```python
from build123d import *

# Parameters (mm, degrees)
SKETCH3_W           = 50
SKETCH3_H           = 50
BOSS_EXTRUDE1_DEPTH = 1.5875
BOSS_EXTRUDE2_DEPTH = 0.204346
SKETCH4_W           = 10
SKETCH4_H           = 10
BOSS_EXTRUDE3_DEPTH = 0.675
SKETCH5_W           = 0.9
SKETCH5_H           = 0.3
BOSS_EXTRUDE4_DEPTH = 0.001


with BuildPart() as part:
    # Sketch3 → Boss-Extrude1 (new body)
    with BuildSketch(Plane(origin=(0, 0, 0), x_dir=(1, 0, 0), z_dir=(0, 1, 0))):
        with Locations((22.488763021, 23.818655395)):
            Rectangle(SKETCH3_W, SKETCH3_H)
    extrude(amount=-BOSS_EXTRUDE1_DEPTH)

    # Sketch2 → Boss-Extrude2 (add)
    with BuildSketch(Plane(origin=(0, 0, 0), x_dir=(1, 0, 0), z_dir=(0, 1, 0))):
        Polygon((32.488763021, 28.302249005), (32.488763021, 40.851579566), (47.488763021, 48.818655395), (-2.511236979, 48.818655395), (12.488763021, 40.851579566), (12.488763021, 28.302249005), align=None)
        Polygon((47.488763021, 31.033343899), (47.488763021, 36.033343899), (42.488763021, 36.033343899), (40.243873607, 34.239185764), (35.010861347, 34.239185764), (35.010861347, 27.818655395), (19.338763021, 27.818655395), (19.338763021, 27.518655395), (36.72925203, 27.518655395), (36.72925203, 32.827502034), (40.243873607, 32.827502034), (42.488763021, 31.033343899), align=None)
        Polygon((47.488763021, -1.181344605), (47.488763021, 3.818655395), (45.72925203, 6.01706342), (45.72925203, 26.536834752), (25.338763021, 26.536834752), (25.338763021, 26.818655395), (25.038763021, 26.818655395), (25.038763021, 26.236834752), (41.093092119, 26.236834752), (44.248274012, 23.081652859), (44.248274012, 6.01706342), (42.488763021, 3.818655395), (42.488763021, -1.181344605), align=None)
        Polygon((33.488763021, -1.181344605), (38.488763021, -1.181344605), (38.488763021, 3.818655395), (36.72925203, 6.01706342), (36.72925203, 24.975395702), (24.138763021, 24.975395702), (24.138763021, 26.818655395), (23.838763021, 26.818655395), (23.838763021, 24.686834752), (33.643092119, 24.686834752), (35.248274012, 23.081652859), (35.248274012, 6.01706342), (33.488763021, 3.818655395), align=None)
        Polygon((24.488763021, 3.818655395), (24.488763021, -1.181344605), (29.488763021, -1.181344605), (29.488763021, 3.818655395), (27.72925203, 6.01706342), (27.72925203, 23.436834752), (22.938763021, 23.436834752), (22.938763021, 26.818655395), (22.638763021, 26.818655395), (22.638763021, 23.136834752), (24.213594494, 23.136834752), (26.248274012, 21.102155233), (26.248274012, 6.01706342), align=None)
        Polygon((15.488763021, 3.818655395), (15.488763021, -1.181344605), (20.488763021, -1.181344605), (20.488763021, 3.818655395), (18.72925203, 6.01706342), (18.731288885, 21.102155233), (20.765968404, 23.136834752), (21.738763021, 23.136834752), (21.738763021, 26.818655395), (21.438763021, 26.818655395), (21.438763021, 23.436834752), (17.248274012, 23.436834752), (17.248274012, 6.01706342), align=None)
        Polygon((6.488763021, 3.818655395), (6.488763021, -1.181344605), (11.488763021, -1.181344605), (11.488763021, 3.818655395), (9.732070762, 6.01706342), (9.732070762, 23.081652859), (11.325813604, 24.686834752), (20.538763021, 24.686834752), (20.538763021, 26.818655395), (20.238763021, 26.818655395), (20.238763021, 24.986834752), (8.24545528, 24.986834752), (8.24545528, 6.01706342), align=None)
        Polygon((-0.735853149, 6.01706342), (-2.511236979, 3.818655395), (-2.511236979, -1.181344605), (2.488763021, -1.181344605), (2.488763021, 3.818655395), (0.729267736, 6.01706342), (0.729267736, 23.081652859), (3.884449629, 26.236834752), (19.338763021, 26.236834752), (19.338763021, 26.818655395), (19.038763021, 26.818655395), (19.038763021, 26.536834752), (-0.735853149, 26.536834752), align=None)
    extrude(amount=BOSS_EXTRUDE2_DEPTH)

    # Sketch4 → Boss-Extrude3 (add)
    with BuildSketch(Plane(origin=(0, 0.204346, 0), x_dir=(1, 0, 0), z_dir=(0, 1, 0))):
        with Locations((22.488763021, 33.818655395)):
            Rectangle(SKETCH4_W, SKETCH4_H)
    extrude(amount=BOSS_EXTRUDE3_DEPTH)

    # Sketch5 → Boss-Extrude4 (add)
    with BuildSketch(Plane(origin=(0, 0.879346, 0), x_dir=(1, 0, 0), z_dir=(0, 1, 0))):
        with Locations((19.488763021, 30.118655395)):
            Rectangle(SKETCH5_W, SKETCH5_H)
        with Locations((20.688763021, 30.118655395)):
            Rectangle(SKETCH5_W, SKETCH5_H)
        with Locations((21.888763021, 30.118655395)):
            Rectangle(SKETCH5_W, SKETCH5_H)
        with Locations((23.088763021, 30.118655395)):
            Rectangle(SKETCH5_W, SKETCH5_H)
        with Locations((24.288763021, 30.118655395)):
            Rectangle(SKETCH5_W, SKETCH5_H)
        with Locations((25.488763021, 30.118655395)):
            Rectangle(SKETCH5_W, SKETCH5_H)
    extrude(amount=BOSS_EXTRUDE4_DEPTH)


solid = part.part
```
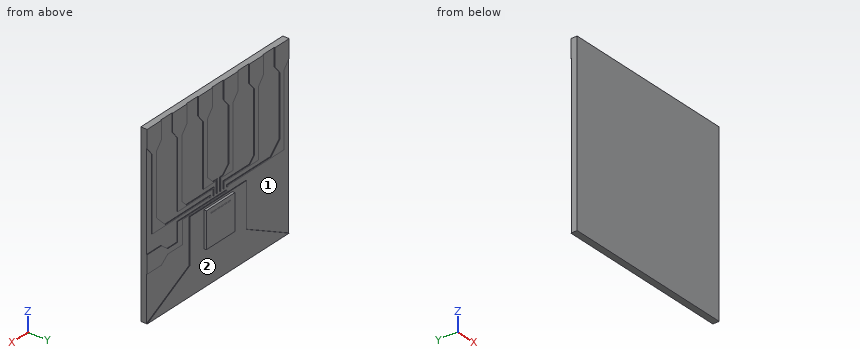
Check sheet for the modelled part. Datum: model origin and axes. Units: mm. Face numbers are marked on the shaded views. Coordinates: 2 decimals unless noted, no trailing zeros. Loops run counter-clockwise (first coordinate to the right, second up) from the corner with the lowest first, then second, coordinate; pieces in that order, holes last. Notation, with made-up numbers: M -25.5,-36 L 0.5,-36 A19 ccw 0.5,-7 Z; hole C 15.25,21.5 d1. An arc over 180 degrees is marked long. Answer as a JSON object with one key per item and string values.
1. Depth check by flat-ended pin: P1, Ø7, axis at x = 13.5, z = -17.5, coming from the +Y side; P2, Ø5.5, axis at x = 25, z = -13, coming from the +Y side; P3, Ø10, axis at x = 25.5, z = -28, coming from the +Y side. Enter the tip coordinate at first touch or a pass-through.
Outcome:
{"P1": "y = 0", "P2": "y = 0.2", "P3": "y = 0.88"}
2. Release check for a two-part mould opening along Z. For the marked faces 1 and 2 record: pulls with the +Z half, pulls with the -Z half, needs draft (parallel to the pull), parting line crosses it, or undercut.
Outcome:
{"face 1": "undercut", "face 2": "needs draft"}
3. Sectioned sample at A-A on x = 37.5. Record the cut outline in (y, z), and give its area (3 significant figures).
Outcome:
{"outline": "M -1.59,-48.82 L 0.2,-48.82 L 0.2,-43.51 L 0,-43.51 L 0,-34.24 L 0.2,-34.24 L 0.2,-32.83 L 0,-32.83 L 0,-26.54 L 0.2,-26.54 L 0.2,-26.24 L 0,-26.24 L 0,-5.05 L 0.2,-5.05 L 0.2,1.18 L -1.59,1.18 Z", "area": "82.1 mm²"}
4. Sectioned sample at B-B on z = -18. Record the cut outline in (x, y), and give its area (3 significant figures).
Outcome:
{"outline": "M -2.51,-1.59 L 47.49,-1.59 L 47.49,0 L 45.73,0 L 45.73,0.2 L 44.25,0.2 L 44.25,0 L 36.73,0 L 36.73,0.2 L 35.25,0.2 L 35.25,0 L 27.73,0 L 27.73,0.2 L 26.25,0.2 L 26.25,0 L 18.73,0 L 18.73,0.2 L 17.25,0.2 L 17.25,0 L 9.73,0 L 9.73,0.2 L 8.25,0.2 L 8.25,0 L 0.73,0 L 0.73,0.2 L -0.74,0.2 L -0.74,0 L -2.51,0 Z", "area": "81.2 mm²"}
5. Scan lines: L1, parallel to X at y = 0.15, z = -13; L2, parallel to Y at x = 23, z = -2.5; L3, parallel to Z at x = 45.5, y = 0.15. Record each from-to range of solid material in increasing order. Write a range as from..to.
Outcome:
{"L1": "-0.74..0.73, 8.25..9.73, 17.25..18.73, 26.25..27.73, 35.25..36.73, 44.25..45.73", "L2": "-1.59..0", "L3": "-48.82..-47.76, -36.03..-31.03, -26.54..1.18"}
6. Sectioned sample at C-C on z = -45.5. Record the cut outline in (x, y), and give its area (3 significant figures).
Outcome:
{"outline": "M -2.51,-1.59 L 47.49,-1.59 L 47.49,0 L 41.24,0 L 41.24,0.2 L 3.74,0.2 L 3.74,0 L -2.51,0 Z", "area": "87.0 mm²"}
